```python
from build123d import *

# Parameters (mm, degrees)
SKETCH2_W          = 728.6625
SKETCH2_H          = 238.125
EXTRUDE1_DEPTH     = 19.05
SKETCH3_R          = 1.5875
SKETCH3_R_2        = 4.7625
SKETCH3_R_3        = 3.175
CUT_EXTRUDE1_DEPTH = 19.05
SKETCH4_W          = 169.8625
SKETCH4_H          = 9.525
CUT_EXTRUDE2_DEPTH = 3.175


with BuildPart() as part:
    # Sketch2 → Extrude1 (new body)
    with BuildSketch(Plane.XY):
        with Locations((-5376.06875, 779.4625)):
            Rectangle(SKETCH2_W, SKETCH2_H)
    extrude(amount=-EXTRUDE1_DEPTH)

    # Sketch3 → Cut-Extrude1 (cut)
    with BuildSketch(Plane.XY):
        with Locations((-5702.3, 892.175)):
            Circle(SKETCH3_R)
        with Locations((-5734.05, 860.425)):
            Circle(SKETCH3_R)
        with Locations((-5713.73, 835.025)):
            Circle(SKETCH3_R_2)
        with Locations((-5712.46, 819.785)):
            Circle(SKETCH3_R_2)
        with Locations((-5712.46, 802.005)):
            Circle(SKETCH3_R_2)
        with Locations((-5712.46, 784.225)):
            Circle(SKETCH3_R_2)
        with Locations((-5734.05, 698.5)):
            Circle(SKETCH3_R)
        with Locations((-5702.3, 666.75)):
            Circle(SKETCH3_R)
        with Locations((-5569.74375, 684.2125)):
            Circle(SKETCH3_R_3)
        with Locations((-5512.59375, 684.2125)):
            Circle(SKETCH3_R_3)
        with Locations((-5474.890625, 666.75)):
            Circle(SKETCH3_R)
        with Locations((-5277.246875, 666.75)):
            Circle(SKETCH3_R)
        with Locations((-5239.54375, 684.2125)):
            Circle(SKETCH3_R_3)
        with Locations((-5182.39375, 684.2125)):
            Circle(SKETCH3_R_3)
        with Locations((-5049.8375, 666.75)):
            Circle(SKETCH3_R)
        with Locations((-5018.0875, 698.5)):
            Circle(SKETCH3_R)
        with Locations((-5018.0875, 860.425)):
            Circle(SKETCH3_R)
        with Locations((-5049.8375, 892.175)):
            Circle(SKETCH3_R)
        with Locations((-5277.246875, 892.175)):
            Circle(SKETCH3_R)
        with Locations((-5474.890625, 892.175)):
            Circle(SKETCH3_R)
        with BuildLine():
            Line((-5291.1375, 803.275), (-5291.1375, 752.475))
            ThreePointArc((-5291.1375, 752.475), (-5287.9625, 749.3), (-5284.7875, 752.475))
            Line((-5284.7875, 752.475), (-5272.0875, 752.475))
            ThreePointArc((-5272.0875, 752.475), (-5268.9125, 749.3), (-5265.7375, 752.475))
            Line((-5265.7375, 752.475), (-5265.7375, 803.275))
            ThreePointArc((-5265.7375, 803.275), (-5268.9125, 806.45), (-5272.0875, 803.275))
            Line((-5272.0875, 803.275), (-5284.7875, 803.275))
            ThreePointArc((-5284.7875, 803.275), (-5287.9625, 806.45), (-5291.1375, 803.275))
        make_face()
    extrude(amount=-CUT_EXTRUDE1_DEPTH, mode=Mode.SUBTRACT)

    # Sketch4 → Cut-Extrude2 (cut)
    with BuildSketch(Plane.XZ.offset(-660.4)):
        with Locations((-5376.06875, -14.2875)):
            Rectangle(SKETCH4_W, SKETCH4_H)
    extrude(amount=-CUT_EXTRUDE2_DEPTH, mode=Mode.SUBTRACT)


solid = part.part
```
CAD build for the part. Positions are in the model's coordinates, mm. A direction names the side the tool comes from. Round coordinates to 2 decimals unless told otherwise and drop trailing zeros. Use a Markdown table: item, result. Add a question column.
(1) Flat gauge pin, fed straight in: pin 1 (5 mm diameter, centred on x = -5335, z = -12.5, fed in from -Y) (3 decimals). Where does the tip first touch, or does it go through?
(2) Which spindle directions (+Z, -Z, +X, -X, +Y, -Y) get a long thin tool onto all of the face, cutting with end or side? Do faces 5 (the face through (-5381, 781, 0)), 6 (the face through (-5279, 752.475, -9)). Say none if no direction does.
(3) Pull direction Y, two halves, no side cores. Call faces 1 (the face through (-5740.4, 778, -9)), 2 (the face through (-5381, 660.4, -9)), 3 (the face through (-5381, 898.525, -9)), 4 (the face through (-5278, 803.275, -9)): +Y half, -Y half, draft (parallel to the pull), parting line (faces both ways), or undercut.
(4) Drill centre lines: line 1 (X direction, y = 861, z = -1); line 2 (X direction, y = 770, z = -13.75); line 3 (X direction, y = 684, z = -8). Where is each one in solid material? Low to high.
Geometry says:
| question | item | result |
|---|---|---|
| 1 | pin 1 | stops at y = 663.575 |
| 2 | face 5 | +Z, +X, -X, +Y, -Y |
| 2 | face 6 | +Z, -Z |
| 3 | face 1 | draft |
| 3 | face 2 | -Y half |
| 3 | face 3 | +Y half |
| 3 | face 4 | undercut |
| 4 | line 1 | x = -5740.4 to -5735.53, -5732.57 to -5019.57, -5016.61 to -5011.74 |
| 4 | line 2 | x = -5740.4 to -5291.14, -5265.74 to -5011.74 |
| 4 | line 3 | x = -5740.4 to -5572.91, -5566.58 to -5515.76, -5509.43 to -5242.71, -5236.38 to -5185.56, -5179.23 to -5011.74 |
